Drawing for the job (mm, zero at the part's lowest x, y, z). A direction names the side the tool comes from. Give positions to 0.01 mm unless a question says otherwise; leave off trailing zeros. Order: outer loops, then holes, each group sorted by start corner. A loop starts at its lowest first (then second) coordinate and runs counter-clockwise, first axis right, second up. Notation, with made-up numbers: M -22,8 L 26,8 A22 ccw 26,38 Z; hole C 77.25,-2.75 d7. An arc over 180 degrees is marked long. One line per item, written item: value.
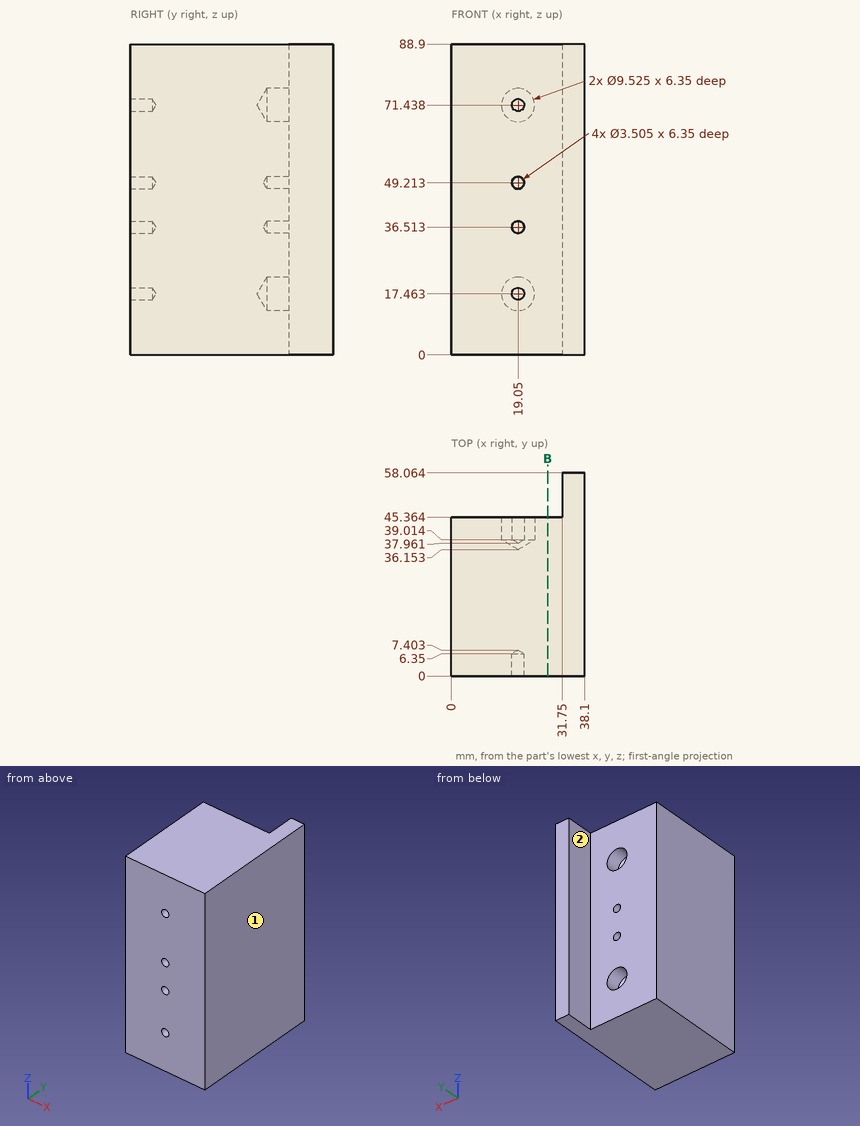
1) Tool access for the marked faces 1 and 2: list every direction of +Z, -Z, +X, -X, +Y, -Y with a clear straight run to the whole face (end or side of a thin tool).
Check values:
face 1: +Z, -Z, +X, +Y, -Y
face 2: +Z, -Z, -X, +Y
2) Pin check, flat tips, straight feed: pin 1 (4.5 mm diameter, centred on x = 19.05, z = 49.21, fed in from +Y); pin 2 (3 mm diameter, centred on x = 19.05, z = 36.51, fed in from +Y) (1 decimal); pin 3 (6.5 mm diameter, centred on y = 55, z = 46.5, fed in from -X). Stop position of each tip, or through.
Check values:
pin 1: y = 45.36
pin 2: y = 38.9
pin 3: x = 31.75
3) Drill centre lines: probe 1 along Z at (x, y) = (19, 5) (1 decimal); probe 2 along Z at (x, y) = (19.05, 41) (1 decimal); probe 3 along Y at (x, z) = (15, 44.5) (1 decimal). Where is each one in solid material? Low to high. Write a range as from..to.
Check values:
probe 1: 0..15.7, 19.2..34.8, 38.3..47.5, 51..69.7, 73.2..88.9
probe 2: 0..12.7, 22.2..34.8, 38.3..47.5, 51..66.7, 76.2..88.9
probe 3: 0..45.4
4) Saw through at B-B, the plane x = 27.5. Write the cut outline in (y, z) (1 decimal), then the cut area to 3 significant figures.
Check values:
outline: M 0,0 L 45.4,0 L 45.4,88.9 L 0,88.9 Z
area: 4,030 mm^2
